Read the model definition and answer for the solid it produces. Units are mm, in the model's axes. Face numbers are marked on the shaded views. A direction names the side the tool comes from. Coordinates: 2 decimals unless noted, no trailing zeros. Order: outer loops, then holes, each group sorted by start corner. A loop starts at its lowest first (then second) coordinate and runs counter-clockwise, first axis right, second up. Notation, with made-up numbers: M -19.75,58 L 2.25,58 A7 ccw 2.25,67 Z; hole C 65,-31 d6. An arc over 180 degrees is marked long. Use a Markdown table: item, result. Add a question column.
1) Find section D-D on z = -6. Write down the section's boundary in (x, y).
2) Find section B-B on y = 2.75. Write down the section's boundary in (x, z).
3) Find the intervals of material crossed by probe 1 along Z at (x, y) = (6.25, 0.75); probe 2 along Z at (x, y) = (11.9, 4); probe 3 along Z at (x, y) = (0, 2), in increasing order. Write a range as [from, to].
4) Find section A-A on x = 0. Write down the section's boundary in (y, z), plus the area to 3 significant figures.
5) For the marked faces 1 and 2, determine the directions among +Z, -Z, +X, -X, +Y, -Y from which every point of the face is accessible in a straight line to the end or side of a thin tool.
6) The mould has two halves that part along Z. Classify the marked faces 3, 4 and 5: released by +Z, released by -Z, zero draft, split by the parting line, or undercut.
7) Find section C-C on z = 0. Write down the section's boundary in (x, y), plus the area to 3 significant figures.
from build123d import *

# Parameters (mm, degrees)
SKETCH1_R           = 1.7
BOSS_EXTRUDE1_DEPTH = 7.5
SKETCH2_R           = 14.5
CUT_EXTRUDE1_DEPTH  = 7.5
SKETCH3_R           = 4
BOSS_EXTRUDE2_DEPTH = 1
BOSS_EXTRUDE3_DEPTH = 1


with BuildPart() as part:
    # Sketch1 → Boss-Extrude1 (new body)
    with BuildSketch(Plane(origin=(0, 0, 0), x_dir=(1, 0, 0), z_dir=(0, 1, 0))):
        with BuildLine():
            Line((-12, -15), (12, -15))
            ThreePointArc((12, -15), (14.121320344, -14.121320344), (15, -12))
            Line((15, -12), (15, 12))
            ThreePointArc((15, 12), (14.121320344, 14.121320344), (12, 15))
            Line((12, 15), (-12, 15))
            ThreePointArc((-12, 15), (-14.121320344, 14.121320344), (-15, 12))
            Line((-15, 12), (-15, -12))
            ThreePointArc((-15, -12), (-14.121320344, -14.121320344), (-12, -15))
        make_face()
        with Locations((-11.9, 11.9)):
            Circle(SKETCH1_R, mode=Mode.SUBTRACT)
        with Locations((11.9, 11.9)):
            Circle(SKETCH1_R, mode=Mode.SUBTRACT)
        with Locations((11.9, -11.9)):
            Circle(SKETCH1_R, mode=Mode.SUBTRACT)
        with Locations((-11.9, -11.9)):
            Circle(SKETCH1_R, mode=Mode.SUBTRACT)
    extrude(amount=BOSS_EXTRUDE1_DEPTH)

    # Sketch2 → Cut-Extrude1 (cut)
    with BuildSketch(Plane(origin=(0, 7.5, 0), x_dir=(1, 0, 0), z_dir=(0, 1, 0))):
        Circle(SKETCH2_R)
    extrude(amount=-CUT_EXTRUDE1_DEPTH, mode=Mode.SUBTRACT)



with BuildPart() as body_2:
    # Sketch3 → Boss-Extrude2 (new body)
    with BuildSketch(Plane.XZ):
        Circle(SKETCH3_R)
    extrude(amount=-BOSS_EXTRUDE2_DEPTH)


with BuildPart() as part_1:
    add(part.part)

    add(body_2.part)  # Boss-Extrude3 merges body 2
    # Sketch4 → Boss-Extrude3 (add)
    with BuildSketch(Plane.XZ):
        with BuildLine():
            Line((-0.5, 14.491376746), (-0.5, 3.968626967))
            ThreePointArc((-0.5, 3.968626967), (0, 4), (0.5, 3.968626967))
            Line((0.5, 3.968626967), (0.5, 14.491376746))
            ThreePointArc((0.5, 14.491376746), (0, 14.5), (-0.5, 14.491376746))
        make_face()
        with BuildLine():
            Line((12.299900398, -7.678701075), (3.186931771, -2.417326185))
            ThreePointArc((3.186931771, -2.417326185), (3.464101615, -2), (3.686931771, -1.551300781))
            Line((3.686931771, -1.551300781), (12.799900398, -6.812675671))
            ThreePointArc((12.799900398, -6.812675671), (12.557368355, -7.25), (12.299900398, -7.678701075))
        make_face()
        with BuildLine():
            Line((-12.799900398, -6.812675671), (-3.686931771, -1.551300781))
            ThreePointArc((-3.686931771, -1.551300781), (-3.464101615, -2), (-3.186931771, -2.417326185))
            Line((-3.186931771, -2.417326185), (-12.299900398, -7.678701075))
            ThreePointArc((-12.299900398, -7.678701075), (-12.557368355, -7.25), (-12.799900398, -6.812675671))
        make_face()
    extrude(amount=-BOSS_EXTRUDE3_DEPTH)


solid = part_1.part
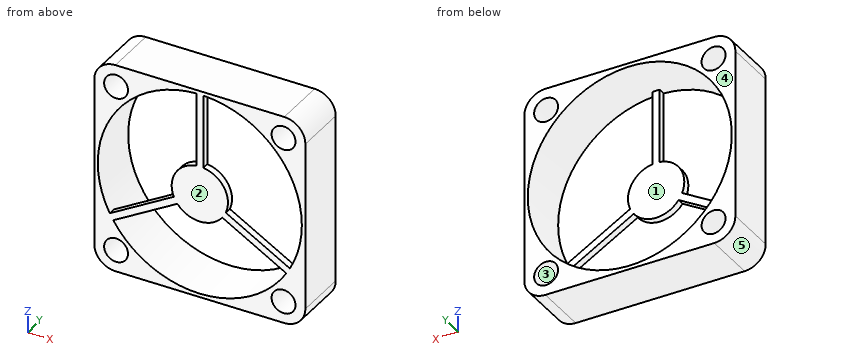
Check result:
| question | item | result |
|---|---|---|
| 1 | outline | M -15,0 L -13.2,0 L -13.2,7.5 L -15,7.5 Z; M -11.39,0 L -9.39,0 L -9.39,1 L -11.39,1 Z; M 9.39,0 L 11.39,0 L 11.39,1 L 9.39,1 Z; M 13.2,0 L 15,0 L 15,7.5 L 13.2,7.5 Z |
| 2 | outline | M -15,-12 A3 ccw -12,-15 L 12,-15 A3 ccw 15,-12 L 15,12 A3 ccw 12,15 L -12,15 A3 ccw -15,12 Z; hole C 0,0 d29; hole C -11.9,-11.9 d3.4; hole C -11.9,11.9 d3.4; hole C 11.9,-11.9 d3.4; hole C 11.9,11.9 d3.4 |
| 3 | probe 1 | z = [-15, -13.08], [-4.19, -3.03], [13.08, 15] |
| 3 | probe 2 | z = [-15, -13.6], [-10.2, -8.28], [8.28, 10.2], [13.6, 15] |
| 3 | probe 3 | z = [-15, -14.5], [14.5, 15] |
| 4 | outline | M 0,-15 L 7.5,-15 L 7.5,-14.5 L 0,-14.5 Z; M 0,-4 L 1,-4 L 1,14.5 L 7.5,14.5 L 7.5,15 L 0,15 Z |
| 4 | area | 26.0 mm2 |
| 5 | face 1 | +Y |
| 5 | face 2 | +Z, -Z, +X, -X, -Y |
| 6 | face 3 | undercut |
| 6 | face 4 | zero draft |
| 6 | face 5 | released by -Z |
| 7 | outline | M -15,0 L -14.5,0 L -14.5,7.5 L -15,7.5 Z; M -4,0 L 4,0 L 4,1 L -4,1 Z; M 14.5,0 L 15,0 L 15,7.5 L 14.5,7.5 Z |
| 7 | area | 15.5 mm2 |
